Autodesk Inventor part; units mm, degrees
ref_plane "YZ Plane" through (0, 0, 0) normal (1, 0, 0) x (0, 1, 0)
ref_plane "XZ Plane" through (0, 0, 0) normal (0, 1, 0) x (-1, 0, 0)
ref_plane "XY Plane" through (0, 0, 0) normal (0, 0, 1) x (1, 0, 0)
sketch "Sketch1" plane through (0, 0, 0) normal (0, 0, 1) x (1, 0, 0)
  line L0 (11, -1) -> (11, 1)
  line L1 (11, 1) -> (-11, 1)
  line L2 (-11, 1) -> (-11, -1)
  line L3 (-11, -1) -> (11, 1) construction
  line L4 (11, -1) -> (-11, 1) construction
  line L5 (11, -1) -> (5.2, -1)
  line L6 (5.2, -1) -> (5.2, -8)
  line L7 (5.2, -8) -> (2.2, -8)
  line L8 (2.2, -8) -> (2.2, -1)
  line L9 (2.2, -1) -> (0, -1)
  line L10 (-10, -2.4556) -> (-3, -2.4556)
  line L11 (-3, -2.4556) -> (-3, -1)
  line L12 (-11, -1) -> (-3, -1)
  line L13 (0, -1) -> (2.2, -1)
  line L14 (5.2, -1) -> (11, -1)
  line L15 (-10, -2.4556) -> (-10, -4.4556)
  line L16 (-10, -4.4556) -> (-8.5, -4.4556)
  line L17 (-8.5, -4.4556) -> (-8.5, -12.4556)
  line L18 (-8.5, -12.4556) -> (-6.5, -12.4556)
  line L19 (-6.5, -12.4556) -> (-6.5, -4.4556)
  line L20 (-6.5, -4.4556) -> (0, -4.4556)
  line L21 (0, -1) -> (0, -4.4556)
  line L22 (5.2, -8) -> (5.7, -8)
  line L23 (5.7, -8) -> (5.7, -6)
  line L24 (5.7, -6) -> (5.2, -6)
  line L25 (5.2, -6) -> (5.2, -8)
  point P0 (0, 0)
  dimension "d0" = 22
  dimension "d1" = 2
  dimension "d2" = 5.8
  dimension "d3" = 7
  dimension "d4" = 3
  dimension "d5" = 2.2
  dimension "d8" = 7
  dimension "d9" = 2
  dimension "d11" = 8
  dimension "d12" = 2
  dimension "d13" = 0.5
  dimension "d14" = 2
extrude "Extrusion1" add sketch "Sketch1" along normal blind 0.5 contours L5 L6 L7 L8 L9 L21 L20 L19 L18 L17 L16 L15 L10 L11 L12 L2 L1 L0
sketch "Sketch2" plane through (0, 0, 0.5) normal (0, 0, 1) x (1, 0, 0)
  line L0 (5.2, -8) -> (5.2, -1)
  line L1 (5.2, -8) -> (5.7, -8)
  line L2 (5.7, -8) -> (5.7, -6)
  line L3 (5.7, -6) -> (5.2, -6)
  line L4 (5.2, -6) -> (5.2, -8)
  point P0 (0, 0)
  point P1 (5.2, -6)
  dimension "d17" = 0.5
  dimension "d18" = 2
extrude "Extrusion2" add sketch "Sketch2" along normal blind 2
sketch "Sketch3" plane through (0, 0, 0.5) normal (0, 0, -1) x (-1, 0, 0)
  line L0 (-5.7, -6) -> (-5.2, -6)
  line L1 (-5.7, -8) -> (-5.7, -6)
  line L2 (-5.2, -8) -> (-5.7, -8)
  line L3 (-5.2, -8) -> (-5.2, -6)
  point P0 (0, 0)
extrude "Extrusion3" add sketch "Sketch3" along normal blind 0.5
sketch "Sketch4" plane through (0, 0, 0.5) normal (0, 0, 1) x (1, 0, 0)
  line L0 (11, 1) -> (-11, 1)
  line L1 (-11, 1) -> (-11, -1)
  line L2 (-11, -1) -> (-3, -1)
  line L3 (-3, -1) -> (-3, -2.4556)
  line L4 (-3, -2.4556) -> (-10, -2.4556)
  line L5 (-10, -2.4556) -> (-10, -4.4556)
  line L6 (-10, -4.4556) -> (-8.5, -4.4556)
  line L7 (-8.5, -4.4556) -> (-8.5, -12.4556)
  line L8 (-8.5, -12.4556) -> (-6.5, -12.4556)
  line L9 (-6.5, -12.4556) -> (-6.5, -4.4556)
  line L10 (-6.5, -4.4556) -> (0, -4.4556)
  line L11 (0, -4.4556) -> (0, -1)
  line L12 (0, -1) -> (2.2, -1)
  line L13 (2.2, -1) -> (2.2, -8)
  line L14 (2.2, -8) -> (5.2, -8)
  line L15 (5.2, -8) -> (5.2, -6)
  line L16 (5.2, -6) -> (5.2, -1)
  line L17 (5.2, -1) -> (11, -1)
  line L18 (11, -1) -> (11, 1)
  line L19 (-3, -1) -> (-3, -2.4556)
  line L20 (0, -1) -> (2.2, -1)
  line L21 (-3, -1) -> (0, -1)
  point P0 (0, 0)
extrude "Extrusion4" add sketch "Sketch4" along normal blind 0.7 contours L21 L11 L10 L9 L8 L7 L6 L5 L4 L3
sketch "Sketch5" plane through (0, 0, 0) normal (0, 0, -1) x (-1, 0, 0)
  line L0 (-11, 1) -> (11, 1)
  line L1 (-11, -1) -> (-11, 1)
  line L2 (-5.2, -1) -> (-11, -1)
  line L3 (-5.2, -6) -> (-5.2, -1)
  line L4 (-5.2, -6) -> (-5.7, -6)
  line L5 (-5.7, -6) -> (-5.7, -8)
  line L6 (-2.2, -8) -> (-5.7, -8)
  line L7 (-2.2, -1) -> (-2.2, -8)
  line L8 (0, -1) -> (-2.2, -1)
  line L9 (0, -4.4556) -> (0, -1)
  line L10 (6.5, -4.4556) -> (0, -4.4556)
  line L11 (6.5, -12.4556) -> (6.5, -4.4556)
  line L12 (8.5, -12.4556) -> (6.5, -12.4556)
  line L13 (8.5, -4.4556) -> (8.5, -12.4556)
  line L14 (10, -4.4556) -> (8.5, -4.4556)
  line L15 (10, -2.4556) -> (10, -4.4556)
  line L16 (3, -2.4556) -> (10, -2.4556)
  line L17 (3, -1) -> (3, -2.4556)
  line L18 (11, -1) -> (3, -1)
  line L19 (11, 1) -> (11, -1)
  line L20 (3, -2.4556) -> (0, -2.4556)
  line L21 (0, -4.4556) -> (0, -1)
  point P0 (0, 0)
extrude "Extrusion5" cut sketch "Sketch5" against normal blind 0.5 contours L16 L15 L14 L13 L12 L11 L10 L9 L20
sketch "Sketch6" plane through (-6.5, -4.4556, 1.2) normal (0, -1, 0) x (1, 0, 0)
  line L0 (6.5, -0.7) -> (6.5, 0)
  line L1 (0, 0) -> (6.5, 0)
  line L2 (6.5, -0.7) -> (0, -0.7)
  line L3 (0, -0.7) -> (0, 0)
  line L4 (0, 0) -> (6.5, 0)
  line L5 (6.5, 0) -> (6.5, -0.7)
  point P0 (6.5, -1.2)
extrude "Extrusion6" add sketch "Sketch6" along normal blind 1.5
sketch "Sketch7" plane through (5.7, -8, 2.5) normal (1, 0, 0) x (0, 0, -1)
  line L0 (0, 2) -> (2.5, 2)
  line L1 (0, 0) -> (0, 2)
  line L2 (2.5, 0) -> (0, 0)
  line L3 (2.5, 2) -> (2.5, 0)
  point P0 (2.5, 8)
extrude "Extrusion7" add sketch "Sketch7" along normal blind 0.5
sketch "Sketch8" plane through (5.2, -8, 0.5) normal (-1, 0, 0) x (0, 0, 1)
  line L0 (0, 0) -> (0, 2)
  line L1 (0, 0) -> (2, 0)
  line L2 (2, 2) -> (2, 0)
  line L3 (0, 2) -> (2, 2)
  point P0 (-0.5, 8)
extrude "Extrusion8" cut sketch "Sketch8" against normal blind 0.5
sketch "Sketch9" plane through (0, 0, 1.2) normal (0, 0, 1) x (1, 0, 0)
  line L0 (-10, -2.4556) -> (-10, -4.4556)
  line L1 (-10, -4.4556) -> (-8.5, -4.4556)
  line L2 (-8.5, -4.4556) -> (-8.5, -12.4556)
  line L3 (-8.5, -12.4556) -> (-6.5, -12.4556)
  line L4 (-6.5, -12.4556) -> (-6.5, -5.9556)
  line L5 (0, -5.9556) -> (-6.5, -5.9556)
  line L6 (0, -1) -> (0, -5.9556)
  line L7 (0, -1) -> (-3, -1)
  line L8 (-3, -1) -> (-3, -2.4556)
  line L9 (-3, -2.4556) -> (-10, -2.4556)
  point P0 (0, 0)
extrude "Extrusion9" cut sketch "Sketch9" against normal blind 0.2
sketch "Sketch10" plane through (0, 0, 0.5) normal (0, 0, -1) x (-1, 0, 0)
  line L0 (6.5, -12.4556) -> (6.5, -5.9556)
  line L1 (8.5, -12.4556) -> (6.5, -12.4556)
  line L2 (8.5, -4.4556) -> (8.5, -12.4556)
  line L3 (10, -4.4556) -> (8.5, -4.4556)
  line L4 (10, -2.4556) -> (10, -4.4556)
  line L5 (3, -2.4556) -> (10, -2.4556)
  line L6 (0, -2.4556) -> (3, -2.4556)
  line L7 (0, -5.9556) -> (0, -2.4556)
  line L8 (6.5, -5.9556) -> (0, -5.9556)
  point P0 (0, 0)
extrude "Extrusion10" add sketch "Sketch10" along normal blind 0.3
sketch "Sketch11" plane through (0, 0, 1) normal (0, 0, 1) x (1, 0, 0)
  line L0 (-3, -2.4556) -> (-3, -1)
  line L1 (-10, -2.4556) -> (-3, -2.4556)
  line L2 (-10, -4.4556) -> (-10, -2.4556)
  line L3 (-8.5, -4.4556) -> (-10, -4.4556)
  line L4 (-8.5, -12.4556) -> (-8.5, -4.4556)
  line L5 (-6.5, -12.4556) -> (-8.5, -12.4556)
  line L6 (-6.5, -5.9556) -> (-6.5, -12.4556)
  line L7 (0, -5.9556) -> (-6.5, -5.9556)
  line L8 (0, -1) -> (0, -5.9556)
  line L9 (-3, -1) -> (0, -1)
  point P0 (0, 0)
extrude "Extrusion11" cut sketch "Sketch11" against normal blind 0.3
sketch "Sketch12" plane through (0, 0, 0.7) normal (0, 0, 1) x (1, 0, 0)
  line L0 (-10, -4.4556) -> (-10, -2.4556)
  line L1 (-8.5, -4.4556) -> (-10, -4.4556)
  line L2 (-8.5, -12.4556) -> (-8.5, -4.4556)
  line L3 (-6.5, -12.4556) -> (-8.5, -12.4556)
  line L4 (-6.5, -5.9556) -> (-6.5, -12.4556)
  line L5 (0, -5.9556) -> (-6.5, -5.9556)
  line L6 (0, -1) -> (0, -5.9556)
  line L7 (-3, -1) -> (0, -1)
  line L8 (-3, -2.4556) -> (-3, -1)
  line L9 (-10, -2.4556) -> (-3, -2.4556)
  point P0 (0, 0)
extrude "Extrusion12" add sketch "Sketch12" along normal blind 0.5
sketch "Sketch13" plane through (0, 0, 0.2) normal (0, 0, -1) x (-1, 0, 0)
  line L0 (8.5, -12.4556) -> (8.5, -4.4556)
  line L1 (8.5, -4.4556) -> (10, -4.4556)
  line L2 (10, -4.4556) -> (10, -2.4556)
  line L3 (10, -2.4556) -> (3, -2.4556)
  line L4 (0, -2.4556) -> (3, -2.4556)
  line L5 (0, -2.4556) -> (0, -5.9556)
  line L6 (0, -5.9556) -> (6.5, -5.9556)
  line L7 (6.5, -5.9556) -> (6.5, -12.4556)
  line L8 (6.5, -12.4556) -> (8.5, -12.4556)
  point P0 (0, 0)
extrude "Extrusion13" cut sketch "Sketch13" against normal blind 0.5
sketch "Sketch14" plane through (6.2, -8, 2.5) normal (1, 0, 0) x (0, 0, -1)
  line L0 (0, 0) -> (2.5, 0)
  line L1 (2.5, 0) -> (2.5, 2)
  line L2 (2.5, 2) -> (0, 2)
  line L3 (0, 2) -> (0, 0)
  point P0 (2.5, 8)
extrude "Extrusion14" add sketch "Sketch14" along normal blind 0.3
sketch "Sketch15" plane through (5.7, -8, 0.5) normal (-1, 0, 0) x (0, 0, 1)
  line L0 (2, 2) -> (2, 0)
  line L1 (0, 2) -> (2, 2)
  line L2 (0, 0) -> (0, 2)
  line L3 (2, 0) -> (0, 0)
  point P0 (-0.5, 8)
extrude "Extrusion15" cut sketch "Sketch15" against normal blind 0.3
sketch "Sketch16" plane through (2.2, -8, 0) normal (-1, 0, 0) x (0, 0, 1)
  line L0 (0, 7) -> (0, 0)
  line L1 (0, 0) -> (0.5, 0)
  line L2 (0.5, 7) -> (0.5, 0)
  line L3 (0, 7) -> (0.5, 7)
  point P0 (0, 8)
extrude "Extrusion16" add sketch "Sketch16" along normal blind 0.04
sketch "Sketch17" plane through (6, -8, 0.5) normal (-1, 0, 0) x (0, 0, 1)
  line L0 (0, 0) -> (0, 2)
  line L1 (2, 0) -> (0, 0)
  line L2 (2, 2) -> (2, 0)
  line L3 (0, 2) -> (2, 2)
  point P0 (-0.5, 8)
extrude "Extrusion17" add sketch "Sketch17" along normal blind 0.125
sketch "Sketch18" plane through (6.5, -8, 2.5) normal (1, 0, 0) x (0, 0, -1)
  line L0 (2.5, 0) -> (2.5, 2)
  line L1 (2.5, 2) -> (0, 2)
  line L2 (0, 2) -> (0, 0)
  line L3 (0, 0) -> (2.5, 0)
  point P0 (2.5, 8)
extrude "Extrusion18" cut sketch "Sketch18" against normal blind 0.125
sketch "Sketch19" plane through (5.2, -1, 0.5) normal (1, 0, 0) x (0, 0, -1)
  line L0 (0, -5) -> (0.5, -5)
  line L1 (0.5, -5) -> (0.5, 0)
  line L2 (0.5, 0) -> (0, 0)
  line L3 (0, -5) -> (0, 0)
  point P0 (0.5, 1)
extrude "Extrusion19" add sketch "Sketch19" along normal blind 1.175
sketch "Sketch20" plane through (5.875, -6, 2.5) normal (0, 1, 0) x (1, 0, 0)
  line L0 (0.5, 2) -> (0, 2)
  line L1 (0, 0) -> (0, 2)
  line L2 (0, 0) -> (0.5, 0)
  line L3 (0.5, 0) -> (0.5, 2)
  point P0 (-5.875, 2.5)
extrude "Extrusion20" add sketch "Sketch20" along normal blind 2
sketch "Sketch21" plane through (2.16, -8, 0) normal (0, -1, 0) x (1, 0, 0)
  line L0 (4.215, 0) -> (4.215, 2.5)
  line L1 (3.715, 2.5) -> (4.215, 2.5)
  line L2 (3.715, 0.5) -> (3.715, 2.5)
  line L3 (3.715, 0.5) -> (0, 0.5)
  line L4 (0, 0) -> (0, 0.5)
  line L5 (4.215, 0) -> (0, 0)
  point P0 (-2.16, 0)
extrude "Extrusion21" cut sketch "Sketch21" against normal blind 1.96
sketch "Sketch22" plane through (5.875, -4, 2.5) normal (0, 1, 0) x (1, 0, 0)
  line L0 (0.5, 0) -> (0.5, 2)
  line L1 (0, 2) -> (0.5, 2)
  line L2 (0, 2) -> (0, 0)
  line L3 (0, 0) -> (0.5, 0)
  point P0 (-5.875, 2.5)
extrude "Extrusion22" cut sketch "Sketch22" against normal blind 1.5
sketch "Sketch23" plane through (2.16, -6.04, 0) normal (0, -1, 0) x (1, 0, 0)
  line L0 (0, 0.5) -> (3.715, 0.5)
  line L1 (4.215, 2.5) -> (4.215, 0)
  line L2 (3.715, 0.5) -> (4.215, 0.5)
  line L3 (4.215, 0.5) -> (4.215, 2.5)
  line L4 (4.215, 2.5) -> (3.715, 2.5)
  line L5 (3.715, 2.5) -> (3.715, 0.5)
  point P0 (-2.16, 0)
extrude "Extrusion23" add sketch "Sketch23" along normal blind 2
sketch "Sketch24" plane through (2.16, -8, 0) normal (-1, 0, 0) x (0, 0, 1)
  line L0 (0, 1.96) -> (0.5, 1.96)
  line L1 (0.5, 1.96) -> (0.5, 7)
  line L2 (0, 7) -> (0.5, 7)
  line L3 (0, 7) -> (0, 1.96)
  point P0 (0, 8)
extrude "Extrusion24" cut sketch "Sketch24" against normal blind 0.75
sketch "Sketch25" plane through (5.875, -8, 0.5) normal (-1, 0, 0) x (0, 0, 1)
  line L0 (2, 2.5) -> (0, 2.5)
  line L1 (0, 1.96) -> (0, 2.5)
  line L2 (0, 1.96) -> (0, -0.04)
  line L3 (2, -0.04) -> (0, -0.04)
  line L4 (2, -0.04) -> (2, 2.5)
  point P0 (-0.5, 8)
extrude "Extrusion25" cut sketch "Sketch25" against normal blind 0.3
sketch "Sketch26" plane through (-8.5, -12.4556, 1.2) normal (-1, 0, 0) x (0, 0, 1)
  line L0 (-0.5, 8) -> (-0.5, 0)
  line L1 (-0.5, 0) -> (0, 0)
  line L2 (0, 8) -> (0, 0)
  line L3 (-0.5, 8) -> (0, 8)
  point P0 (-1.2, 12.4556)
extrude "Extrusion26" add sketch "Sketch26" along normal blind 0.5
properties part number "TerminalR"
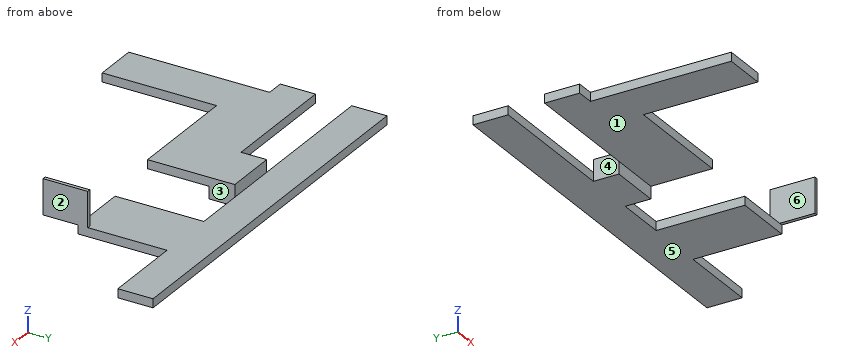
Geometry check sheet. Reference: the model listing, model coordinates, mm. Face numbers are marked on the shaded views. A direction names the side the tool comes from. Round coordinates to 2 decimals unless told otherwise and drop trailing zeros. Loops run counter-clockwise (first coordinate to the right, second up) from the corner with the lowest first, then second, coordinate; pieces in that order, holes last. Notation, with made-up numbers: (-7.5, -5) - (1.5, -5) arc R14 ccw to (1.5, 22) - close; hole circle Ø2 at (25.25, 69). An arc over 180 degrees is marked (long way). Write each question's results on one line, items separated by ' | '. Start each with the question number.
Q1. Cross-section at C-C on x = -2.5. Enter the section's corners in (y, z).
Q2. Release check for a two-part mould opening along X. For the marked faces 1, 2 and 3 record: +X half, -X half, draft (parallel to the pull), parting line (faces both ways), or undercut.
Q3. Cross-section at A-A on y = -4. Enter the section's corners in (x, z) (3 decimals).
Q4. Gauge pin test, flat ends, axial feed: P1, Ø1, axis at x = -0.5, z = 1, coming from the -Y side; P2, Ø1.2, axis at y = -5, z = 1, coming from the +X side (3 decimals); P3, Ø5, axis at x = -5.5, y = -8, coming from the -Z side. Record the tip position at first contact, or that the pin passes through.
Q5. Cross-section at D-D on z = 1.45. Enter the section's corners in (x, y) (3 decimals), and give its area (3 significant figures).
Q6. Cross-section at B-B on x = -7.25. Enter the section's corners in (y, z).
Q7. Access from +Z, -Z, +X, -X, +Y, -Y to the whole of each face (thin tool, end or side, straight path). Record for the marked faces 4, 5 and 6.
Q8. Thickness scan on line 1 (Z direction, x = 5.5, y = -2.25); line 2 (Z direction, x = -5.5, y = -3); line 3 (Y direction, x = -5.75, z = 0.45). Record the ranges inside material, lowest first. Write a range as [from, to].
Answers below:
1) outline: (-5.96, 0.7) - (-2.46, 0.7) - (-2.46, 0) - (1, 0) - (1, 0.5) - (-1, 0.5) - (-1, 1.2) - (-5.96, 1.2) - close
2) face 1: draft | face 2: +X half | face 3: undercut
3) outline: (-10, 0.7) - (0, 0.7) - (0, 1.2) - (-10, 1.2) - close; (2.91, 0) - (6.375, 0) - (6.375, 0.5) - (2.91, 0.5) - close
4) P1: stops at y = -5.96 | P2: stops at x = 6.375 | P3: stops at z = 0.7
5) outline: (6.175, -8.04) - (6.375, -8.04) - (6.375, -5.5) - (6.175, -5.5) - close | area: 0.508 mm²
6) outline: (-12.46, 0.7) - (-2.46, 0.7) - (-2.46, 1.2) - (-12.46, 1.2) - close; (-1, 0) - (1, 0) - (1, 0.5) - (-1, 0.5) - close
7) face 4: +Z, -Z, -X | face 5: -Z, +X, -X, +Y, -Y | face 6: +Z, +Y, -Y
8) line 1: z = [0, 0.5] | line 2: z = [0.7, 1.2] | line 3: y = [-1, 1]
